```python
from build123d import *

# Parameters (mm, degrees)
SKETCH1_W           = 6
SKETCH1_H           = 19
SKETCH1_W_2         = 8
SKETCH1_H_2         = 10
BOSS_EXTRUDE1_DEPTH = 4
BOSS_EXTRUDE2_DEPTH = 3
BOSS_EXTRUDE3_START = -3
BOSS_EXTRUDE3_DEPTH = 3
SKETCH6_R           = 1
CUT_EXTRUDE1_DEPTH  = 14
SKETCH7_R           = 1
CUT_EXTRUDE2_DEPTH  = 14


with BuildPart() as part:
    # Sketch1 → Boss-Extrude1 (new body)
    with BuildSketch(Plane(origin=(0, 0, 0), x_dir=(1, 0, 0), z_dir=(0, 1, 0))):
        with Locations((3, 9.5)):
            Rectangle(SKETCH1_W, SKETCH1_H)
        with Locations((-4, 9.5)):
            Rectangle(SKETCH1_W_2, SKETCH1_H_2)
    extrude(amount=BOSS_EXTRUDE1_DEPTH)

    # Sketch2 → Boss-Extrude2 (add)
    with BuildSketch(Plane.XY.offset(-4.5)):
        with BuildLine():
            Line((-8, 0), (-10, 0))
            ThreePointArc((-10, 0), (-12, 2), (-10, 4))
            Line((-10, 4), (-8, 4))
            Line((-8, 4), (-8, 0))
        make_face()
    extrude(amount=-BOSS_EXTRUDE2_DEPTH)

    # Sketch5 → Boss-Extrude3 (add)
    with BuildSketch(Plane(origin=(0, 0, -14.5), x_dir=(-1, 0, 0), z_dir=(0, 0, -1)).offset(BOSS_EXTRUDE3_START)):
        with BuildLine():
            Line((8, 4), (10, 4))
            ThreePointArc((10, 4), (12, 2), (10, 0))
            Line((10, 0), (8, 0))
            Line((8, 0), (8, 4))
        make_face()
    extrude(amount=BOSS_EXTRUDE3_DEPTH)

    # Sketch6 → Cut-Extrude1 (cut)
    with BuildSketch(Plane(origin=(0, 0, -14.5), x_dir=(-1, 0, 0), z_dir=(0, 0, -1))):
        with Locations((10.127972383, 2)):
            Circle(SKETCH6_R)
    extrude(amount=-CUT_EXTRUDE1_DEPTH, mode=Mode.SUBTRACT)

    # Sketch7 → Cut-Extrude2 (cut)
    with BuildSketch(Plane(origin=(0, 0, -14.5), x_dir=(-1, 0, 0), z_dir=(0, 0, -1))):
        with Locations((4, 2)):
            Circle(SKETCH7_R)
    extrude(amount=-CUT_EXTRUDE2_DEPTH, mode=Mode.SUBTRACT)


solid = part.part
```
Check sheet for the modelled part. Datum: model origin and axes. Units: mm. A direction names the side the tool comes from. Round coordinates to 2 decimals unless told otherwise and drop trailing zeros. Loops run counter-clockwise (first coordinate to the right, second up) from the corner with the lowest first, then second, coordinate; pieces in that order, holes last. Notation, with made-up numbers: (-10.75, -15) -> (1.25, -15) arc R34 cw to (1.25, 15) -> close; hole circle Ø11 at (21.5, -15.75). An arc over 180 degrees is marked (long way). Write item = value, one per line. Start each with the question number.
1) Sectioned sample at A-A, the plane x = -4. Record the cut outline in (y, z).
2) Sectioned sample at B-B, the plane y = 2. Record the cut outline in (x, z), plus the area to 3 significant figures.
3) Set-up check for faces 5 (the flat face through (0, 2, -2)), 6 (the flat face through (-8.7, 2, -11.5)), 7 (the flat face through (0, 2, -17)), 8 (the cylindrical face through (-3.2, 1.4, -9.6)): record each of +Z, -Z, +X, -X, +Y, -Y from which the full face is reachable in a straight line by a thin tool's end or side.
4) Sectioned sample at D-D, the plane y = 3.3. Record the cut outline in (x, z).
5) Gauge pin test, flat ends, axial feed: pin 1 Ø1.2 at (x, y) = (-8.5, 2) entering from -Z; pin 2 Ø1.8 at (x, y) = (-10.13, 2) entering from -Z; pin 3 Ø1.5 at (x, y) = (1, 2) entering from +Z; pin 4 Ø2 at (x, y) = (-5.5, 1.5) entering from +Z. Record the tip position at first contact, or that the pin passes through.
6) Sectioned sample at C-C, the plane x = -9.5. Record the cut outline in (y, z).
7) Release check for a two-part mould opening along Z. For faces 1 (the flat face through (3, 2, -19)), 2 (the cylindrical face through (-11.08, 2.3, -13.02)), 3 (the flat face through (-9, 1, -7.5)), 4 (the flat face through (-8, 2, -9)) record: released by +Z, released by -Z, zero draft, split by the parting line, or undercut.
8) Thickness scan on probe 1 along X at (y, z) = (2.3, -5); probe 2 along X at (y, z) = (3, -2.5); probe 3 along X at (y, z) = (0.95, -10). Record the ranges inside material, lowest first.
Results are:
q1.outline = (0, -14.5) -> (1, -14.5) -> (1, -4.5) -> (0, -4.5) -> close; (3, -14.5) -> (4, -14.5) -> (4, -4.5) -> (3, -4.5) -> close
q2.outline = (-12, -14.5) -> (-11.13, -14.5) -> (-11.13, -11.5) -> (-12, -11.5) -> close; (-12, -7.5) -> (-11.13, -7.5) -> (-11.13, -4.5) -> (-12, -4.5) -> close; (-9.13, -14.5) -> (-5, -14.5) -> (-5, -4.5) -> (-9.13, -4.5) -> (-9.13, -7.5) -> (-8, -7.5) -> (-8, -11.5) -> (-9.13, -11.5) -> close; (-3, -14.5) -> (0, -14.5) -> (0, -19) -> (6, -19) -> (6, 0) -> (0, 0) -> (0, -4.5) -> (-3, -4.5) -> close
q2.area = 186 mm^2
q3.face_5 = +Z, -X, +Y, -Y
q3.face_6 = -X, +Y, -Y
q3.face_7 = -Z, -X, +Y, -Y
q3.face_8 = +Z, -Z
q4.outline = (-11.52, -14.5) -> (0, -14.5) -> (0, -19) -> (6, -19) -> (6, 0) -> (0, 0) -> (0, -4.5) -> (-11.52, -4.5) -> (-11.52, -7.5) -> (-8, -7.5) -> (-8, -11.5) -> (-11.52, -11.5) -> close
q5.pin_1 = -14.5
q5.pin_2 = through
q5.pin_3 = 0
q5.pin_4 = -4.5
q6.outline = (0, -14.5) -> (1.22, -14.5) -> (1.22, -11.5) -> (0, -11.5) -> close; (0, -7.5) -> (1.22, -7.5) -> (1.22, -4.5) -> (0, -4.5) -> close; (2.78, -14.5) -> (4, -14.5) -> (4, -11.5) -> (2.78, -11.5) -> close; (2.78, -7.5) -> (4, -7.5) -> (4, -4.5) -> (2.78, -4.5) -> close
q7.face_1 = released by -Z
q7.face_2 = zero draft
q7.face_3 = undercut
q7.face_4 = undercut
q8.probe_1 = -11.98 to -11.08, -9.17 to -4.95, -3.05 to 6
q8.probe_2 = 0 to 6
q8.probe_3 = -8 to 6
